```python
from build123d import *

# Parameters (mm, degrees)
SKETCH58_R          = 1
BOSS_EXTRUDE1_DEPTH = 6.464
SKETCH59_W          = 2.864
SKETCH59_H          = 0.3
FILLET6_R           = 0.5
FILLET7_R           = 0.3
SKETCH54_R          = 0.25


with BuildPart() as part:
    # Sketch58 → Boss-Extrude1 (new body)
    with BuildSketch(Plane(origin=(0, 0, 0), x_dir=(0, 0, -1), z_dir=(1, 0, 0))):
        Circle(SKETCH58_R)
    extrude(amount=BOSS_EXTRUDE1_DEPTH)

    # Sketch59 → Cut-Revolve1 (revolve, cut)
    with BuildSketch(Plane.XY, mode=Mode.PRIVATE) as cut_revolve1_sk:
        with Locations((3.232, 1)):
            Rectangle(SKETCH59_W, SKETCH59_H)
    revolve(cut_revolve1_sk.sketch.rotate(Axis((6.464, 0, 0), (-1, 0, 0)), 90), axis=Axis((6.464, 0, 0), (-1, 0, 0)), mode=Mode.SUBTRACT)

    # Fillet6
    # the kernel refuses this fillet: 0.5 mm, written as the material it takes off along each edge
    with BuildSketch(Plane(origin=(0, 0, 0), x_dir=(0, 0, -1), z_dir=(0, -1, 0))) as fillet6_piece_1:
        with BuildLine():
            CenterArc((1 - FILLET6_R, FILLET6_R), FILLET6_R, 270, 90)
            Line((1 - FILLET6_R, 0), (1 - FILLET6_R, -FILLET6_R * 0.02))
            Line((1 - FILLET6_R, -FILLET6_R * 0.02), (1 + FILLET6_R * 0.02, -FILLET6_R * 0.02))
            Line((1 + FILLET6_R * 0.02, -FILLET6_R * 0.02), (1 + FILLET6_R * 0.02, FILLET6_R))
            Line((1 + FILLET6_R * 0.02, FILLET6_R), (1, FILLET6_R))
        make_face()
    revolve(axis=Axis((0, 0, 0), (1, 0, 0)), mode=Mode.SUBTRACT)
    with BuildSketch(Plane(origin=(6.464, 0, 0), x_dir=(0, 0, -1), z_dir=(0, -1, 0))) as fillet6_piece_2:
        with BuildLine():
            CenterArc((1 - FILLET6_R, -FILLET6_R), FILLET6_R, 0, 90)
            Line((1 - FILLET6_R, 0), (1 - FILLET6_R, FILLET6_R * 0.02))
            Line((1 - FILLET6_R, FILLET6_R * 0.02), (1 + FILLET6_R * 0.02, FILLET6_R * 0.02))
            Line((1 + FILLET6_R * 0.02, FILLET6_R * 0.02), (1 + FILLET6_R * 0.02, -FILLET6_R))
            Line((1 + FILLET6_R * 0.02, -FILLET6_R), (1, -FILLET6_R))
        make_face()
    revolve(axis=Axis((6.464, 0, 0), (1, 0, 0)), mode=Mode.SUBTRACT)
    with BuildSketch(Plane(origin=(1.8, 0, 0), x_dir=(0, 0, -1), z_dir=(0, 1, 0))) as fillet6_piece_3:
        with BuildLine():
            CenterArc((0.5, 0.357071421), FILLET6_R, 314.427004001, 45.572995999)
            Line((0.85, 0), (0.857, -0.007141428))
            ThreePointArc((0.857, -0.007141428), (0.925, -0.01), (1, -0.01))
            Line((1, -0.01), (1.01, 0))
            Line((1.01, 0), (1.01, 0.357071421))
            Line((1.01, 0.357071421), (1, 0.357071421))
        make_face()
    revolve(axis=Axis((1.8, 0, 0), (-1, 0, 0)), mode=Mode.SUBTRACT)
    with BuildSketch(Plane(origin=(4.664, 0, 0), x_dir=(0, 0, -1), z_dir=(0, 1, 0))) as fillet6_piece_4:
        with BuildLine():
            CenterArc((0.5, -0.357071421), FILLET6_R, 0, 45.572995999)
            Line((1, -0.357071421), (1.01, -0.357071421))
            Line((1.01, -0.357071421), (1.01, 0))
            Line((1.01, 0), (1, 0.01))
            ThreePointArc((1, 0.01), (0.925, 0.01), (0.857, 0.007141428))
            Line((0.857, 0.007141428), (0.85, 0))
        make_face()
    revolve(axis=Axis((4.664, 0, 0), (-1, 0, 0)), mode=Mode.SUBTRACT)

    # Fillet7
    fillet7_edges = [part.edges().sort_by_distance(p)[0] for p in [
        (1.8, 0, 0.85),
        (4.664, 0, 0.85),
    ]]
    fillet(fillet7_edges, radius=FILLET7_R)

    # Sweep1: sweep along a path in Sketch55
    with BuildLine(Plane.XY) as sweep1_path:
        Line((0, 0), (-0.2, 0))
        ThreePointArc((-0.2, 0), (-0.907106781, -0.292893219), (-1.2, -1))
        Line((-1.2, -1), (-1.2, -6))
    # Sketch54 → Sweep1 (sweep)
    with BuildSketch(Plane(origin=(0, 0, 0), x_dir=(0, 0, -1), z_dir=(1, 0, 0))):
        Circle(SKETCH54_R)
    sweep1 = sweep(path=sweep1_path.line)

    # Mirror1: Sweep1 across plane
    add(sweep1.mirror(Plane(origin=(3.232, 0, 0), x_dir=(0, 0, 1), z_dir=(1, 0, 0))))


solid = part.part
```
Here's how the part is built. I have some questions about the finished solid (model axes, mm). Coordinates: 2 decimals unless noted, no trailing zeros. Loops run counter-clockwise (first coordinate to the right, second up) from the corner with the lowest first, then second, coordinate; pieces in that order, holes last. Notation, with made-up numbers: (61, -13) - (77, -13) arc R31 cw to (77, 15) - close; hole circle Ø4 at (51.5, -19). An arc over 180 degrees is marked (long way). Return JSON: item names as keys, results as strings. Group by question number.
Item 1: I need wall thicknesses on line 1 (X direction, y = -1.25, z = 0); line 2 (X direction, y = -0.25, z = 0.35); line 3 (X direction, y = -0.5, z = -0.8). Which ranges of each line are inside material? Lowest first, please. Write a range as from..to.
Item 2: If we section it at A-A on y = -5: Write out the boundary of the cut face in (x, z), and give its area (3 significant figures).
Item 3: Will this pin go through, and if not, where does the flat tip stop? P1, Ø0.5, axis at y = 0, z = 0, coming from the +X side.
Calculated:
{
 "1": {"line 1": "x = -1.45..-0.95, 7.41..7.91", "line 2": "x = 0..6.46", "line 3": "x = 0.27..1.67, 4.79..6.2"},
 "2": {"outline": "circle Ø0.5 at (-1.2, 0); circle Ø0.5 at (7.66, 0)", "area": "0.393 mm^2"},
 "3": {"P1": "stops at x = 7.66"}
}
